Source: CAD feature listing. Evaluate the final solid. Frame: model axes, mm. A direction names the side the tool comes from. Give positions to 0.01 mm unless a question says otherwise; leave off trailing zeros. Loops run counter-clockwise (first coordinate to the right, second up) from the corner with the lowest first, then second, coordinate; pieces in that order, holes last. Notation, with made-up numbers: (25.25, 40) -> (70.25, 40) arc R16 cw to (70.25, 61) -> close; hole circle Ø2 at (44, 2). An arc over 180 degrees is marked (long way). Return JSON: item names as keys, results as strings. Group by question number.
```python
from build123d import *

# Parameters (mm, degrees)
CUT_EXTRUDE_START         = -1.5
CUT_EXTRUDE_1_OUTLINE_W   = 9
CUT_EXTRUDE_1_OUTLINE_H   = 6
CUT_EXTRUDE_1_DEPTH       = 0.7
CUT_EXTRUDE_START_2       = 0.8
CUT_EXTRUDE_1_2_OUTLINE_W = 9
CUT_EXTRUDE_1_2_OUTLINE_H = 6
CUT_EXTRUDE_1_2_DEPTH     = 0.7
CUT_EXTRUDE_2_DEPTH       = 8.431016081
CUT_EXTRUDE_2_DEPTH_BACK  = 8.431016081
SKETCH_4_R                = 0.55
CUT_EXTRUDE_3_DEPTH       = 9.766413178
CUT_EXTRUDE_3_DEPTH_BACK  = 1
SKETCH_5_OUTSIDE_W        = 6.85
SKETCH_5_OUTSIDE_H        = 5.45
SKETCH_5_OUTSIDE_W_2      = 0.6
SKETCH_5_OUTSIDE_H_2      = 3.351666402
SKETCH_7_R                = 0.3
CUT_EXTRUDE_5_DEPTH       = 8.368174808


# Read off the part's stored shape, not the designer's step: 切除-拉伸1
with BuildPart() as part:
    # 草图2 → 旋转1 (revolve)
    with BuildSketch(Plane(origin=(0, 0, 0), x_dir=(1, 0, 0), z_dir=(0, 1, 0)), mode=Mode.PRIVATE) as revolve_1_sk:
        with BuildLine():
            ThreePointArc((1.5, 0), (1.388672279, 0.567088443), (1.071214264, 1.05))
            ThreePointArc((1.071214264, 1.05), (-0.567088443, 1.388672279), (-1.5, 0))
            Line((-1.5, 0), (1.5, 0))
        make_face()
        with BuildLine():
            Line((3.5, 1.05), (1.071214264, 1.05))
            ThreePointArc((1.071214264, 1.05), (1.388672279, 0.567088443), (1.5, 0))
            Line((1.5, 0), (7.1, 0))
            Line((7.1, 0), (7.1, 0.6))
            Line((7.1, 0.6), (5.1, 0.6))
            Line((5.1, 0.6), (3.5, 1.05))
        make_face()
    revolve(revolve_1_sk.sketch.rotate(Axis((7.1, 0, 0), (1, 0, 0)), 180), axis=Axis((7.1, 0, 0), (1, 0, 0)))

    # 切除-拉伸1 outline → 切除-拉伸1 (cut)
    with BuildSketch(Plane(origin=(0, 0, 0), x_dir=(1, 0, 0), z_dir=(0, 1, 0)).offset(CUT_EXTRUDE_START)):
        with Locations((1.5, 0)):
            Rectangle(CUT_EXTRUDE_1_OUTLINE_W, CUT_EXTRUDE_1_OUTLINE_H)
    extrude(amount=CUT_EXTRUDE_1_DEPTH, mode=Mode.SUBTRACT)

    # Cut-Extrude 1 2 outline → Cut-Extrude 1 2 (cut)
    with BuildSketch(Plane(origin=(0, 0, 0), x_dir=(1, 0, 0), z_dir=(0, 1, 0)).offset(CUT_EXTRUDE_START_2)):
        with Locations((1.5, 0)):
            Rectangle(CUT_EXTRUDE_1_2_OUTLINE_W, CUT_EXTRUDE_1_2_OUTLINE_H)
    extrude(amount=CUT_EXTRUDE_1_2_DEPTH, mode=Mode.SUBTRACT)

    # 草图4 → 切除-拉伸2 (cut, two sides: drawn at the far end of the back side and taken through both)
    with BuildSketch(Plane(origin=(0, 0.8, 0), x_dir=(1, 0, 0), z_dir=(0, 1, 0)).offset(-CUT_EXTRUDE_2_DEPTH_BACK)):
        with Locations(Location((0, 0, 0), (0, 0, 270))):
            Circle(SKETCH_4_R)
    extrude(amount=CUT_EXTRUDE_2_DEPTH + CUT_EXTRUDE_2_DEPTH_BACK, mode=Mode.SUBTRACT)

    # 草图5 outside → 切除-拉伸3 (cut, two sides: drawn at the far end of the back side and taken through both)
    with BuildSketch(Plane(origin=(7.1, 0, 0), x_dir=(0, 0, -1), z_dir=(1, 0, 0)).offset(-CUT_EXTRUDE_3_DEPTH_BACK)):
        Rectangle(SKETCH_5_OUTSIDE_W, SKETCH_5_OUTSIDE_H)
        Rectangle(SKETCH_5_OUTSIDE_W_2, SKETCH_5_OUTSIDE_H_2, mode=Mode.SUBTRACT)
    extrude(amount=CUT_EXTRUDE_3_DEPTH + CUT_EXTRUDE_3_DEPTH_BACK, mode=Mode.SUBTRACT)

    # 草图7 → 切除-拉伸5 (cut, through all)
    with BuildSketch(Plane(origin=(0, 0, -0.3), x_dir=(-1, 0, 0), z_dir=(0, 0, -1))):
        with Locations((-6.6, 0)):
            Circle(SKETCH_7_R)
    extrude(amount=-CUT_EXTRUDE_5_DEPTH, mode=Mode.SUBTRACT)


solid = part.part
```
1) Cut plane D-D on x = 0. Return loops of the section in (y, z).
2) Contact query for a flat-ended pin moving along its axis: P1, Ø0.5, axis at x = 6.5, y = 0, coming from the -Z side. Output: stop coordinate, or through.
3) Reachability of faces 1 (the face through (2.27, 0.01, 1.05)), 2 (the face through (5.86, 0.53, 0.28)), 3 (the face through (2.27, -0.01, -1.05)) from +Z, -Z, +X, -X, +Y, -Y: full face, straight path, thin tool, end or side. Return the list, or none.
4) Cut plane B-B on z = 0. Return loops of the section in (x, y).
5) Cut plane C-C on x = 6.6. Return loops of the section in (y, z).
6) Material intervals for line 1 (X direction, y = -0.15, z = 0); line 2 (Y direction, x = 6.6, z = -0.05); line 3 (Z direction, x = 0, y = 0.15), sorted ascending.
7) Cut plane A-A on y = 0. Return loops of the section in (x, z), then the cut area to 3 significant figures.
Calculated:
{
 "1": {"outline": "(-0.8, -1.27) arc R1.5 ccw to (0.8, -1.27) -> (0.8, -0.55) -> (-0.8, -0.55) -> close; (-0.8, 0.55) -> (0.8, 0.55) -> (0.8, 1.27) arc R1.5 ccw to (-0.8, 1.27) -> close"},
 "2": {"P1": "z = -0.3"},
 "3": {"face 1": "+Z, +X", "face 2": "+X", "face 3": "-Z, +X"},
 "4": {"outline": "(-1.27, -0.8) -> (-0.55, -0.8) -> (-0.55, 0.8) -> (-1.27, 0.8) arc R1.5 ccw to start; (0.55, -0.8) -> (4.39, -0.8) -> (5.1, -0.6) -> (7.1, -0.6) -> (7.1, 0.6) -> (5.1, 0.6) -> (4.39, 0.8) -> (0.55, 0.8) -> close; hole circle Ø0.6 at (6.6, 0)"},
 "5": {"outline": "(-0.52, -0.3) -> (-0.3, -0.3) -> (-0.3, 0.3) -> (-0.52, 0.3) arc R0.6 ccw to start; (0.3, -0.3) -> (0.52, -0.3) arc R0.6 ccw to (0.52, 0.3) -> (0.3, 0.3) -> close"},
 "6": {"line 1": "-1.49 to -0.55, 0.55 to 6.34, 6.86 to 7.1", "line 2": "-0.6 to -0.3, 0.3 to 0.6", "line 3": "-1.49 to -0.55, 0.55 to 1.49"},
 "7": {"outline": "(1.07, -1.05) -> (3.5, -1.05) -> (5.1, -0.6) -> (6.1, -0.6) -> (6.1, -0.3) -> (6.3, -0.3) -> (6.3, 0.3) -> (6.1, 0.3) -> (6.1, 0.6) -> (5.1, 0.6) -> (3.5, 1.05) -> (1.07, 1.05) arc R1.5 ccw (long way) to start; (6.9, -0.3) -> (7.1, -0.3) -> (7.1, 0.3) -> (6.9, 0.3) -> close; hole circle Ø1.1 at (0, 0)", "area": "14.7 mm2"}
}
